Input: part model. Units: mm. Frame: model coordinates. A direction names the side the tool comes from. Coordinates: 2 decimals unless noted, no trailing zeros. Order: outer loops, then holes, each group sorted by start corner. A loop starts at its lowest first (then second) coordinate and runs counter-clockwise, first axis right, second up. Notation, with made-up numbers: M -34.5,-5 L -6.5,-5 A18 ccw -6.5,23 Z; hole C 45.25,2.25 d9. An arc over 180 degrees is marked long. One line per item, written item: value.
Autodesk Inventor part; units mm, degrees
ref_plane "YZ Plane" through (0, 0, 0) normal (1, 0, 0) x (0, 1, 0)
ref_plane "XZ Plane" through (0, 0, 0) normal (0, 1, 0) x (-1, 0, 0)
ref_plane "XY Plane" through (0, 0, 0) normal (0, 0, 1) x (1, 0, 0)
sketch "Esquisse1" plane through (0, 0, 0) normal (0, 1, 0) x (-1, 0, 0)
  line L0 (0, 0) -> (40.8419, 40.8419) construction
  line L1 (0, 0) -> (43.2459, 0) construction
  line L2 (0, 0) -> (0, 37.214) construction
  line L3 (31.4289, 0) -> (31.4289, 10)
  line L4 (31.4289, 10) -> (38.5, 17.0711)
  line L5 (38.5, 17.0711) -> (27.7855, 27.7855)
  line L6 (0, 31.4289) -> (10, 31.4289)
  line L7 (10, 31.4289) -> (17.0711, 38.5)
  line L8 (17.0711, 38.5) -> (27.7855, 27.7855)
  line L9 (31.4289, 0) -> (31.4289, -10)
  line L10 (31.4289, -10) -> (38.5, -17.0711)
  line L11 (38.5, -17.0711) -> (27.7855, -27.7855)
  line L12 (0, -31.4289) -> (10, -31.4289)
  line L13 (10, -31.4289) -> (17.0711, -38.5)
  line L14 (17.0711, -38.5) -> (27.7855, -27.7855)
  line L15 (0, 0) -> (-40.8419, 40.8419) construction
  line L16 (0, 0) -> (-43.2459, 0) construction
  line L17 (-31.4289, 0) -> (-31.4289, 10)
  line L18 (-31.4289, 10) -> (-38.5, 17.0711)
  line L19 (-38.5, 17.0711) -> (-27.7855, 27.7855)
  line L20 (0, 31.4289) -> (-10, 31.4289)
  line L21 (-10, 31.4289) -> (-17.0711, 38.5)
  line L22 (-17.0711, 38.5) -> (-27.7855, 27.7855)
  line L23 (-38.5, -17.0711) -> (-27.7855, -27.7855)
  line L24 (-31.4289, -10) -> (-38.5, -17.0711)
  line L25 (-31.4289, 0) -> (-31.4289, -10)
  line L26 (-17.0711, -38.5) -> (-27.7855, -27.7855)
  line L27 (-10, -31.4289) -> (-17.0711, -38.5)
  line L28 (0, -31.4289) -> (-10, -31.4289)
  dimension "d4" = 45
  dimension "d5" = 10
  dimension "d6" = 10
  dimension "d7" = 38.5
  dimension "d10" = 77
extrude "Extrusion1" add sketch "Esquisse1" along normal blind 1.6
sketch "Esquisse3" plane through (0, 0, 0) normal (0, -1, 0) x (1, 0, 0)
  line L0 (-31.4289, -10) -> (-31.4289, 10) construction
  line L1 (-38.5, -17.0711) -> (-31.4289, -10) construction
  line L2 (-17.0711, -38.5) -> (-38.5, -17.0711) construction
  line L3 (-10, -31.4289) -> (-17.0711, -38.5) construction
  line L4 (10, -31.4289) -> (-10, -31.4289) construction
  line L5 (17.0711, -38.5) -> (10, -31.4289) construction
  line L6 (38.5, -17.0711) -> (17.0711, -38.5) construction
  line L7 (31.4289, -10) -> (38.5, -17.0711) construction
  line L8 (31.4289, 10) -> (31.4289, -10) construction
  line L9 (38.5, 17.0711) -> (31.4289, 10) construction
  line L10 (17.0711, 38.5) -> (38.5, 17.0711) construction
  line L11 (10, 31.4289) -> (17.0711, 38.5) construction
  line L12 (-10, 31.4289) -> (10, 31.4289) construction
  line L13 (-17.0711, 38.5) -> (-10, 31.4289) construction
  line L14 (-38.5, 17.0711) -> (-17.0711, 38.5) construction
  line L15 (-31.4289, 10) -> (-38.5, 17.0711) construction
  circle A0 centre (-32.136, 17.0711) radius 1.75
  circle A1 centre (-17.0711, -32.136) radius 1.75
  circle A2 centre (32.136, -17.0711) radius 1.75
  circle A3 centre (17.0711, 32.136) radius 1.75
  point P0 (0, 0)
  point P1 (16, 32)
  point P2 (0, 0)
  point P3 (0, 0)
  point P4 (0, 0)
  dimension "d36" = 4.5
  dimension "d37" = 4.5
  dimension "d38" = 3.5
  dimension "d41" = 360
extrude "Extrusion2" cut sketch "Esquisse3" against normal through all
sketch "Esquisse4" plane through (0, 0, 0) normal (0, -1, 0) x (1, 0, 0)
  point P0 (0, 0)
sketch "Esquisse5" plane through (0, 0, 0) normal (0, -1, 0) x (1, 0, 0)
  line L0 (-31.4289, -10) -> (-31.4289, 10) construction
  line L1 (-38.5, -17.0711) -> (-31.4289, -10) construction
  line L2 (-17.0711, -38.5) -> (-38.5, -17.0711) construction
  line L3 (-10, -31.4289) -> (-17.0711, -38.5) construction
  line L4 (10, -31.4289) -> (-10, -31.4289) construction
  line L5 (17.0711, -38.5) -> (10, -31.4289) construction
  line L6 (38.5, -17.0711) -> (17.0711, -38.5) construction
  line L7 (31.4289, -10) -> (38.5, -17.0711) construction
  line L8 (31.4289, 10) -> (31.4289, -10) construction
  line L9 (38.5, 17.0711) -> (31.4289, 10) construction
  line L10 (17.0711, 38.5) -> (38.5, 17.0711) construction
  line L11 (10, 31.4289) -> (17.0711, 38.5) construction
  line L12 (-10, 31.4289) -> (10, 31.4289) construction
  line L13 (-17.0711, 38.5) -> (-10, 31.4289) construction
  line L14 (-38.5, 17.0711) -> (-17.0711, 38.5) construction
  line L15 (-31.4289, 10) -> (-38.5, 17.0711) construction
  line L16 (0, 0) -> (-31.4289, 0) construction
  line L17 (0, 0) -> (0, -31.4289) construction
  dimension "d29" = 38.5
  dimension "d30" = 17.0711
  dimension "d31" = 31.4289
  dimension "d32" = 10
  dimension "d33" = 17.0711
  dimension "d34" = 38.5
  dimension "d35" = 10
sketch "Esquisse6" plane through (0, 0, 0) normal (0, -1, 0) x (1, 0, 0)
  line L0 (22.0329, 30.7097) -> (-14.2473, -5.5705)
  line L1 (-14.2473, -5.5705) -> (-1.3158, -18.5021)
  line L2 (-1.3158, -18.5021) -> (34.9645, 17.7782)
  line L3 (34.9645, 17.7782) -> (22.0329, 30.7097)
  line L4 (17.0711, 38.5) -> (38.5, 17.0711)
  line L5 (38.5, 17.0711) -> (31.4289, 10)
  point P0 (0, 0)
  dimension "d43" = 2
  dimension "d44" = 51.308
  dimension "d45" = 18.288
  dimension "d46" = 3
extrude "Extrusion3" add sketch "Esquisse6" along normal blind 10
sketch "Esquisse7" plane through (0, -10, 0) normal (0, -1, 0) x (1, 0, 0)
  line L0 (21.4276, 22.8297) -> (27.0845, 17.1729)
  line L1 (27.0845, 17.1729) -> (31.3271, 21.4155)
  line L2 (31.3271, 21.4155) -> (25.6703, 27.0724)
  line L3 (25.6703, 27.0724) -> (21.4276, 22.8297)
  line L4 (34.9645, 17.7782) -> (22.0329, 30.7097)
  point P0 (0, 0)
  point P1 (28.4987, 24.244)
  dimension "d49" = 8
  dimension "d50" = 6
extrude "Extrusion4" add sketch "Esquisse7" along normal blind 4
properties part number "x_board"
(1) Access query for faces 4 (the flat face through (-34.915, 0.789, -13.486)), 5 (the flat face through (13.486, 0.789, -34.915)), 6 (the flat face through (34.915, 0.789, -13.486)). Directions: +Z, -Z, +X, -X, +Y, -Y. A direction counts if a zero-diameter tool reaches every point of the face in a straight line with its end or side. Return the directions, or none.
Data:
face 4: -X, +Y, -Y
face 5: -Z, +Y, -Y
face 6: +X, +Y, -Y
(2) Cut plane C-C on x = 6. Output: boundary loops of the cut face in (y, z), plus the area to 3 significant figures.
Data:
outline: M -10,-11.19 L 0,-11.19 L 0,-31.43 L 1.6,-31.43 L 1.6,31.43 L 0,31.43 L 0,14.68 L -10,14.68 Z
area: 359 mm2
(3) Cut plane D-D on y = -5.75. Output: boundary loops of the cut face in (x, z).
Data:
outline: M -14.25,-5.57 L -1.32,-18.5 L 34.96,17.78 L 22.03,30.71 Z
(4) Cut plane A-A on z = -7.5. Output: boundary loops of the cut face in (x, y).
Data:
outline: M -31.43,0 L -12.32,0 L -12.32,-10 L 9.69,-10 L 9.69,0 L 31.43,0 L 31.43,1.6 L -31.43,1.6 Z
(5) Cut plane B-B on y = -12.5. Output: boundary loops of the cut face in (x, z).
Data:
outline: M 21.43,22.83 L 27.08,17.17 L 31.33,21.42 L 25.67,27.07 Z
(6) Draft query along Z for faces 1 (the flat face through (-34.915, 0.789, 13.486)), 2 (the flat face through (16.57, -4.93, -0.616)), 3 (the flat face through (23.6, -12, 25)). Return one class per face: released by +Z, released by -Z, zero draft, split by the parting line, or undercut.
Data:
face 1: undercut
face 2: released by -Z
face 3: released by +Z
(7) Ray query, line 1 (Y direction, x = -23, z = 19); line 2 (Z direction, x = 6, y = 1.25); line 3 (Y direction, x = 22, z = 10). Return the intervals inside material, ascending. Write a range as from..to.
Data:
line 1: y = 0..1.6
line 2: z = -31.43..31.43
line 3: y = -10..1.6
(8) First-contact query: pin 1 (2 mm diameter, centred on y = -2, z = 3.5, fed in from -X); pin 2 (1.8 mm diameter, centred on x = -3, y = 1, fed in from -Z); pin 3 (1 mm diameter, centred on x = -18.5, z = 25.5, fed in from -Y). Flat tips, straight axial feed; report the tip coordinate or a pass-through.
Data:
pin 1: stops at x = -6.18
pin 2: stops at z = -31.43
pin 3: stops at y = 0
